from build123d import *


with BuildPart() as part:
    # Sketch1 → Revolve1 (revolve)
    with BuildSketch(Plane.XY, mode=Mode.PRIVATE) as revolve1_sk:
        Polygon((-2.38125, 3.3655), (-2.19075, 3.175), (2.19075, 3.175), (2.38125, 3.3655), (2.38125, 4.191), (1.190625, 4.191), (1.190625, 5.7404), (1.741289063, 5.7404), (1.741289063, 4.6101), (1.830585938, 4.6101), (1.830585938, 5.7404), (2.38125, 5.7404), (2.38125, 6.085416667), (2.116666667, 6.35), (-2.116666667, 6.35), (-2.38125, 6.085416667), (-2.38125, 5.7404), (-1.830585937, 5.7404), (-1.830585937, 4.6101), (-1.741289062, 4.6101), (-1.741289062, 5.7404), (-1.190625, 5.7404), (-1.190625, 4.191), (-2.38125, 4.191), align=None)
    revolve(revolve1_sk.sketch.rotate(Axis((-2.38125, 0, 0), (1, 0, 0)), 270), axis=Axis((-2.38125, 0, 0), (1, 0, 0)))


solid = part.part
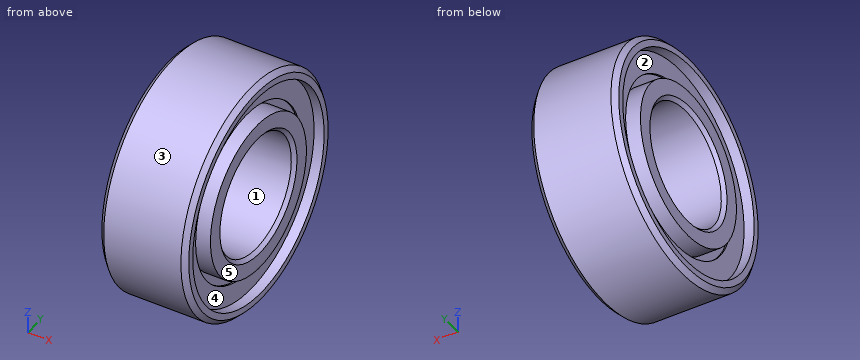
The listing builds one solid part. Answer for the finished solid, in the listing's coordinates (mm). Face numbers are marked on the shaded views. A direction names the side the tool comes from. Round coordinates to 2 decimals unless told otherwise and drop trailing zeros. Order: outer loops, then holes, each group sorted by start corner. A loop starts at its lowest first (then second) coordinate and runs counter-clockwise, first axis right, second up. Notation, with made-up numbers: (-10.75, 69) -> (19.25, 69) arc R26 ccw to (19.25, 88) -> close; hole circle Ø3 at (75.5, -10.5). An arc over 180 degrees is marked (long way). Write each question's results on one line, items separated by ' | '. Start each with the question number.
Q1. The mould has two halves that part along Y. Classify the marked faces 3, 4 and 5: pulls with the +Y half, pulls with the -Y half, needs draft (parallel to the pull), parting line crosses it, or undercut.
Q2. Each of these flat-tipped pins is pushed along its axis until it touches: pin 1 (1 mm diameter, centred on x = 2, z = 5, fed in from +Y); pin 2 (1.5 mm diameter, centred on x = 1.5, z = 1.5, fed in from +Y); pin 3 (1.5 mm diameter, centred on x = 1, y = 4, fed in from +Z); pin 4 (1.5 mm diameter, centred on y = 0.5, z = 1.5, fed in from +X). Where does it stop, or does it pass through?
Q3. Find section B-B (z = -5.5). Give the number of separate pieces and of enclosed holes in the cut face, then the cut area to 3 significant figures.
Q4. Straight lines are drawn through the part: probe 1 along Y at (x, z) = (-1.25, 0) (3 decimals); probe 2 along Y at (x, z) = (1.7, -0.5); probe 3 along Z at (x, y) = (1.55, 2.25). For each, find the intervals that lie inside material, in ascending order. Write a range as from..to.
Q5. Find section A-A (x = 0.2). Determine the outline of the cut face in (y, z) (3 decimals).
Q6. Which of the six approach directions +Z, -Z, +X, -X, +Y, -Y give full straight-line access (tool end or side, diameter ignored) to the marked faces 1 and 2?
Worked answers:
1) face 3: parting line crosses it | face 4: undercut | face 5: needs draft
2) pin 1: stops at y = 4.48 | pin 2: stops at y = 6.31 | pin 3: stops at z = 5.46 | pin 4: passes through
3) separate pieces: 1 | enclosed holes: 2 | area: 22.7 mm2
4) probe 1: y = -6.35..-5.74, -4.191..-3.175, 3.175..4.191, 5.74..6.35 | probe 2: y = -6.33..-5.72, -4.16..-3.14, 3.14..4.16, 5.72..6.33 | probe 3: z = -5.94..-5.28, -3.54..-2.24, 2.24..3.54, 5.28..5.94
5) outline: circle Ø12.7 at (0, 0); hole circle Ø6.35 at (0, 0)
6) face 1: +X, -X | face 2: -X
